```python
from build123d import *

# Parameters (mm, degrees)
BOSS_EXTRUDE2_DEPTH = 152.4


with BuildPart() as part:
    # Sketch2 → Boss-Extrude2 (new body, symmetric)
    with BuildSketch(Plane.XY):
        with BuildLine():
            Line((0, 0), (0, 177.8))
            Line((0, 177.8), (0.00508, 177.8))
            ThreePointArc((0.00508, 177.8), (8.981744019, 174.081744019), (12.7, 165.10508))
            Line((12.7, 165.10508), (12.7, 25.4))
            ThreePointArc((12.7, 25.4), (16.419743879, 16.419743879), (25.4, 12.7))
            Line((25.4, 12.7), (88.90508, 12.7))
            ThreePointArc((88.90508, 12.7), (97.881744019, 8.981744019), (101.6, 0.00508))
            Line((101.6, 0.00508), (101.6, 0))
            Line((101.6, 0), (0, 0))
        make_face()
    extrude(amount=BOSS_EXTRUDE2_DEPTH, both=True)


solid = part.part
```
Read the model definition and answer for the solid it produces. Units are mm, in the model's axes. A direction names the side the tool comes from. Coordinates: 2 decimals unless noted, no trailing zeros. Write each loop counter-clockwise with the first axis right and the second up, starting at its lowest first coordinate (ties: lowest second). Pieces come first, ordered by that corner, then holes. Notation, with made-up numbers: (-29.5, 60.5) -> (-14.5, 60.5) arc R24 ccw to (-14.5, 72.5) -> close; hole circle Ø9 at (59.25, 1). An arc over 180 degrees is marked (long way). Write item = value, one per line.
(1) Section B-B on x = 47 is taken. Write down the section's boundary in (y, z).
From the geometry:
outline = (0, -152.4) -> (12.7, -152.4) -> (12.7, 152.4) -> (0, 152.4) -> close
(2) Straight lines are drawn through the part: L1, parallel to Y at x = 67.5, z = -26.5; L2, parallel to Y at x = 96, z = 48.5. For each, find the intervals that lie inside material, in ascending order. Write a range as from..to.
From the geometry:
L1 = 0..12.7
L2 = 0..10.53
(3) Which of the six approach directions +Z, -Z, +X, -X, +Y, -Y give full straight-line access (tool end or side, diameter ignored) to faces 1 (the face through (57, 12.7, 2)), 2 (the face through (0, 88, 2))?
From the geometry:
face_1 = +Z, -Z, +X, +Y
face_2 = +Z, -Z, -X, +Y, -Y
(4) Given pin 1 Ø1.5 at (y, z) = (71, 16) entering from +X; pin 2 Ø12 at (x, y) = (21, 64.5) entering from +Z; pin 3 Ø19 at (x, z) = (47.5, 52) entering from +Y; pin 4 Ø10 at (x, z) = (25, -94.5) entering from +Y, each flat-ended and moving along its own axis, determine where each tip first touches the part or whether it passes through.
From the geometry:
pin_1 = 12.7
pin_2 = through
pin_3 = 12.7
pin_4 = 13.91
